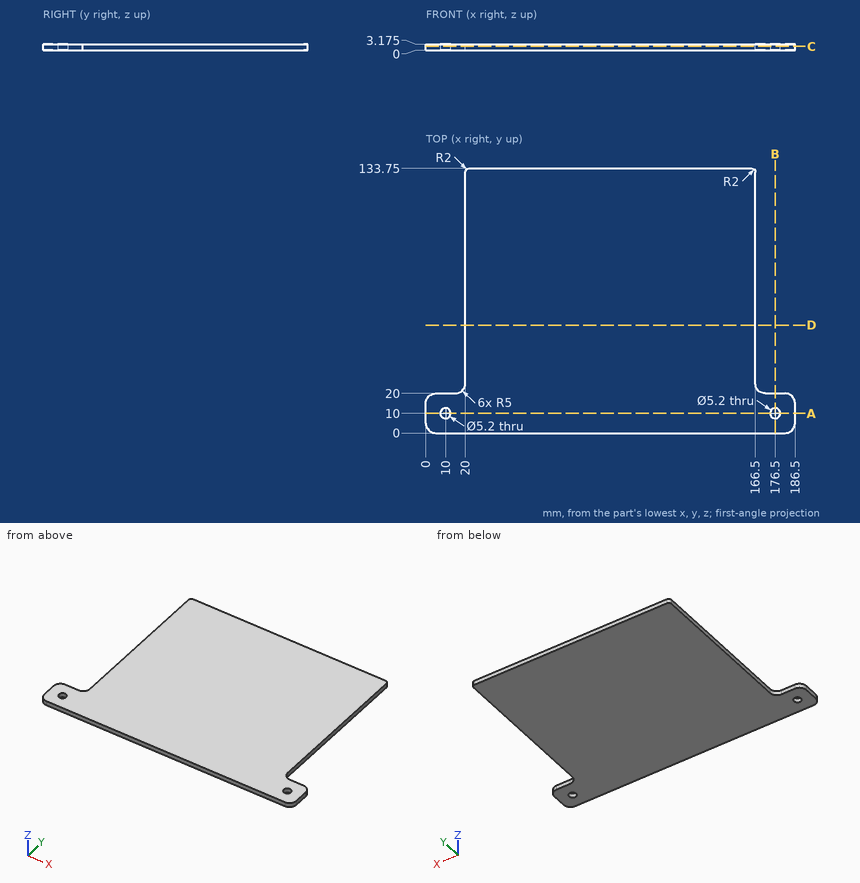
Can you work these out from the drawing? Everything is in mm from the part's minimum corner. Round coordinates to 2 decimals unless told otherwise and drop trailing zeros. Write each loop counter-clockwise with the first axis right and the second up, starting at its lowest first coordinate (ties: lowest second). Pieces come first, ordered by that corner, then holes. Notation, with made-up numbers: (88.25, 27.25) - (103.25, 27.25) arc R32 cw to (103.25, 61.25) - close; hole circle Ø8 at (56, -34). An arc over 180 degrees is marked (long way). Use a Markdown table: item, result.
Q1. I want a section at B-B (x = 176.5). List the corners of the cut face in (y, z) for me (3 decimals).
Output values:
| item | result |
|---|---|
| outline | (0, 0) - (7.4, 0) - (7.4, 3.175) - (0, 3.175) - close; (12.6, 0) - (20, 0) - (20, 3.175) - (12.6, 3.175) - close |
Q2. Please list where these lines run through material, in increasing order: L1, parallel to Y at x = 176.5, z = 1.75; L2, parallel to X at y = 101.5, z = 0.65.
Output values:
| item | result |
|---|---|
| L1 | 0 to 7.4, 12.6 to 20 |
| L2 | 20 to 166.5 |
Q3. For pin 1 (1 mm diameter, centred on y = 99, z = 2, fed in from +X); pin 2 (1.6 mm diameter, centred on y = 104.5, z = 2.5, fed in from -X); pin 3 (1 mm diameter, centred on x = 11, z = 2.5, fed in from +Y), each with a flat end and sliding along its axis, tell me the tip position at first contact or that it passes through.
Output values:
| item | result |
|---|---|
| pin 1 | x = 166.5 |
| pin 2 | x = 20 |
| pin 3 | y = 20 |
Q4. I want a section at A-A (y = 10). List the corners of the cut face in (x, z) for me (3 decimals).
Output values:
| item | result |
|---|---|
| outline | (0, 0) - (7.4, 0) - (7.4, 3.175) - (0, 3.175) - close; (12.6, 0) - (173.9, 0) - (173.9, 3.175) - (12.6, 3.175) - close; (179.1, 0) - (186.5, 0) - (186.5, 3.175) - (179.1, 3.175) - close |
Q5. I want a section at C-C (z = 1.95). List the corners of the cut face in (x, y) for me, plus the area to 3 significant figures.
Output values:
| item | result |
|---|---|
| outline | (0, 5) arc R5 ccw to (5, 0) - (181.5, 0) arc R5 ccw to (186.5, 5) - (186.5, 15) arc R5 ccw to (181.5, 20) - (171.5, 20) arc R5 cw to (166.5, 25) - (166.5, 131.75) arc R2 ccw to (164.5, 133.75) - (22, 133.75) arc R2 ccw to (20, 131.75) - (20, 25) arc R5 cw to (15, 20) - (5, 20) arc R5 ccw to (0, 15) - close; hole circle Ø5.2 at (10, 10); hole circle Ø5.2 at (176.5, 10) |
| area | 20,300 mm2 |
Q6. I want a section at D-D (y = 54.5). List the corners of the cut face in (x, z) for me (3 decimals), plus the area to 3 significant figures.
Output values:
| item | result |
|---|---|
| outline | (20, 0) - (166.5, 0) - (166.5, 3.175) - (20, 3.175) - close |
| area | 465 mm2 |
